```python
from build123d import *

# Parameters (mm, degrees)
SKETCH1_W           = 97
SKETCH1_H           = 83
BOSS_EXTRUDE1_DEPTH = 4
FILLET1_R           = 4
SKETCH3_R           = 1.25
CUT_EXTRUDE1_DEPTH  = 10
CUT_EXTRUDE2_DEPTH  = 2
SKETCH5_W           = 2
SKETCH5_H           = 25
CUT_EXTRUDE3_DEPTH  = 10
LPATTERN1_COUNT     = 10
LPATTERN1_PITCH     = 5
SKETCH6_R           = 3
CUT_EXTRUDE4_DEPTH  = 105


with BuildPart() as part:
    # Sketch1 → Boss-Extrude1 (new body)
    with BuildSketch(Plane(origin=(0, 0, 0), x_dir=(1, 0, 0), z_dir=(0, 1, 0))):
        with Locations((3.439716312, -14.541223404)):
            Rectangle(SKETCH1_W, SKETCH1_H)
    extrude(amount=BOSS_EXTRUDE1_DEPTH)

    # Fillet1
    fillet1_edges = [part.edges().sort_by_distance(p)[0] for p in [
        (3.439716312, 4, -26.958776596),
        (51.939716312, 4, 14.541223404),
        (3.439716312, 4, 56.041223404),
        (-45.060283688, 4, 14.541223404),
    ]]
    fillet(fillet1_edges, radius=FILLET1_R - 0.0001)  # a hair under: the kernel refuses the full size

    # Sketch3 → Cut-Extrude1 (cut)
    with BuildSketch(Plane.XZ):
        with Locations(Location((-42.560283688, 40.041223404, 0), (0, 0, 270))):
            Circle(SKETCH3_R)
        with Locations(Location((49.439716312, 40.041223404, 0), (0, 0, 270))):
            Circle(SKETCH3_R)
        with Locations(Location((-42.560283688, -10.958776596, 0), (0, 0, 270))):
            Circle(SKETCH3_R)
        with Locations(Location((49.439716312, -10.958776596, 0), (0, 0, 270))):
            Circle(SKETCH3_R)
    extrude(amount=-CUT_EXTRUDE1_DEPTH, mode=Mode.SUBTRACT)

    # Sketch4 → Cut-Extrude2 (cut)
    with BuildSketch(Plane(origin=(0, 4, 0), x_dir=(1, 0, 0), z_dir=(0, 1, 0))):
        with BuildLine():
            Line((-42.560283688, 13.458776596), (-49.206472021, 13.458776596))
            Line((-49.206472021, 13.458776596), (-49.206472021, 8.458776596))
            Line((-49.206472021, 8.458776596), (-42.560283688, 8.458776596))
            ThreePointArc((-42.560283688, 8.458776596), (-40.060283688, 10.958776596), (-42.560283688, 13.458776596))
        make_face()
        with BuildLine():
            Line((-42.560283688, -37.541223404), (-49.554151242, -37.541223404))
            Line((-49.554151242, -37.541223404), (-49.554151242, -42.541223404))
            Line((-49.554151242, -42.541223404), (-42.560283688, -42.541223404))
            ThreePointArc((-42.560283688, -42.541223404), (-40.060283688, -40.041223404), (-42.560283688, -37.541223404))
        make_face()
        with BuildLine():
            Line((49.439716312, 13.458776596), (53.973660089, 13.458776596))
            Line((53.973660089, 13.458776596), (53.973660089, 8.458776596))
            Line((53.973660089, 8.458776596), (49.439716312, 8.458776596))
            ThreePointArc((49.439716312, 8.458776596), (46.939716312, 10.958776596), (49.439716312, 13.458776596))
        make_face()
        with BuildLine():
            Line((49.439716312, -37.541223404), (55.815990307, -37.541223404))
            Line((55.815990307, -37.541223404), (55.815990307, -42.541223404))
            Line((55.815990307, -42.541223404), (49.439716312, -42.541223404))
            ThreePointArc((49.439716312, -42.541223404), (46.939716312, -40.041223404), (49.439716312, -37.541223404))
        make_face()
    extrude(amount=-CUT_EXTRUDE2_DEPTH, mode=Mode.SUBTRACT)

    # Sketch5 → Cut-Extrude3 (cut)
    with BuildSketch(Plane(origin=(0, 4, 0), x_dir=(1, 0, 0), z_dir=(0, 1, 0))):
        with Locations((-19.060283688, 2.958776596)):
            Rectangle(SKETCH5_W, SKETCH5_H)
        with Locations((-19.060283688, -32.041223404)):
            Rectangle(SKETCH5_W, SKETCH5_H)
    cut_extrude3 = extrude(amount=-CUT_EXTRUDE3_DEPTH, mode=Mode.SUBTRACT)

    # LPattern1: Cut-Extrude3 ×10
    with Locations(*[(i * LPATTERN1_PITCH, 0, 0) for i in range(1, LPATTERN1_COUNT)]):
        add(cut_extrude3, mode=Mode.SUBTRACT)

    # Sketch6 → Cut-Extrude4 (cut)
    with BuildSketch(Plane(origin=(0, 4, 0), x_dir=(1, 0, 0), z_dir=(0, 1, 0))):
        with Locations(Location((38.066563645, -14.541223404, 0), (0, 0, 270))):
            Circle(SKETCH6_R)
    extrude(amount=-CUT_EXTRUDE4_DEPTH, mode=Mode.SUBTRACT)


solid = part.part
```
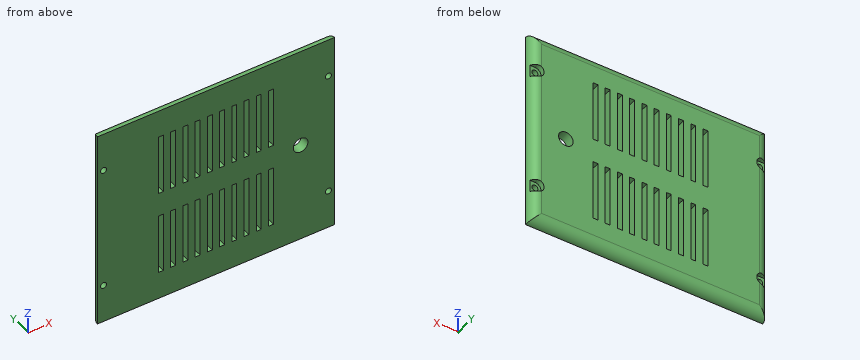
Verification items for the finished model (mm, model axes). Give positions to 0.01 mm unless a question says otherwise; leave off trailing zeros. Answer as CSV lines item,"result". Start each with the question number.
Item 1: Gauge pin test, flat ends, axial feed: pin 1 (1 mm diameter, centred on x = -2, y = 2.5, fed in from +Z); pin 2 (2 mm diameter, centred on y = 1.5, z = -8, fed in from +X); pin 3 (2 mm diameter, centred on x = 6.5, y = 2.5, fed in from +Z); pin 4 (1 mm diameter, centred on x = 13.5, z = 34.5, fed in from -Y). Record the tip position at first contact, or that the pin passes through.
Item 2: Section check A-A, the plane z = -7. State how many separate pieces and enclosed holes the cut face has, plus the area to 3 significant figures.
Item 3: Material ranges on L1, parallel to Z at x = 10, y = 1.3; L2, parallel to Z at x = 11, y = 2.75; L3, parallel to X at y = 2.7, z = 17, recorded low to high.
Filled in:
1,pin 1,"z = 55.51"
1,pin 2,"x = 51.91"
1,pin 3,"z = 55.75"
1,pin 4,"y = 0"
2,separate pieces,"11"
2,enclosed holes,"0"
2,area,"301 mm^2"
3,L1,"-26.74 to -15.46, 9.54 to 19.54, 44.54 to 55.82"
3,L2,"-25.86 to -15.46, 9.54 to 19.54, 44.54 to 54.95"
3,L3,"-44.01 to 36.35, 39.79 to 50.89"
